Autodesk Inventor part; units mm, degrees
ref_plane "YZ Plane" through (0, 0, 0) normal (1, 0, 0) x (0, 1, 0)
ref_plane "XZ Plane" through (0, 0, 0) normal (0, 1, 0) x (-1, 0, 0)
ref_plane "XY Plane" through (0, 0, 0) normal (0, 0, 1) x (1, 0, 0)
sketch "Sketch1" plane through (0, 0, 0) normal (0, 0, 1) x (1, 0, 0)
  arc A0 (-37, 0) -> (37, 0) centre (0, 0) ccw
  line L0 (-51.8, 0) -> (51.8, 0) construction
  circle A1 centre (0, 0) radius 35 construction
  line L1 (-37, 0) -> (37, 0)
  dimension "d1" = 70
  dimension "d2" = 2
extrude "Extrusion1" add sketch "Sketch1" along normal blind 2
sketch "Sketch2" plane through (0, 0, 2) normal (0, 0, 1) x (1, 0, 0)
  arc A0 (-37, 0) -> (37, 0) centre (0, 0) ccw
  arc A1 (-35, 0) -> (35, 0) centre (0, 0) ccw
  line L0 (37, 0) -> (-37, 0)
  line L1 (-37, 0) -> (37, 0)
  dimension "d5" = 2
extrude "Extrusion2" add sketch "Sketch2" along normal blind 35 contours L0 A1 A0
ref_plane "Work Plane1" through (0, 0, 19.5) normal (0, 0, 1) x (1, 0, 0)
mirror "Mirror1" about plane through (0, 0, 19.5) normal (0, 0, 1) of "Extrusion1"
sketch "Sketch3" plane through (0, 0, 39) normal (0, 0, 1) x (1, 0, 0)
  circle A0 centre (0, 0) radius 21
  dimension "d8" = 42
extrude "Extrusion3" cut sketch "Sketch3" against normal blind 35
sketch "Sketch4" plane through (0, 0, 0) normal (1, 0, 0) x (0, 1, 0)
  line L0 (-4, 9.5) -> (-31, 9.5)
  line L1 (-31, 9.5) -> (-31, 29.5)
  line L2 (-31, 29.5) -> (-4, 29.5)
  line L3 (-4, 29.5) -> (-4, 9.5)
  line L4 (-44.4, 19.5) -> (7.4, 19.5) construction
  line L5 (0, 0) -> (0, 39) construction
  line L6 (-35, 37) -> (-35, 2) construction
  dimension "d11" = 20
  dimension "d12" = 4
  dimension "d13" = 4
extrude "Extrusion4" cut sketch "Sketch4" along normal through all both and the other way through all
sketch "Sketch5" plane through (0, 0, 0) normal (0, 1, 0) x (-1, 0, 0)
  line L0 (37, 0) -> (-37, 0)
  line L1 (0, -31.0583) -> (0, 50.6764) construction
  line L2 (-6, -3) -> (6, -3)
  line L3 (6, -3) -> (6, -5.2)
  line L4 (6, -5.2) -> (-6, -5.2)
  line L5 (-6, -5.2) -> (-6, -3)
  line L6 (-2.5, -5.2) -> (2.5, -5.2)
  line L7 (2.5, -5.2) -> (2.5, -11.2)
  line L8 (2.5, -11.2) -> (-2.5, -11.2)
  line L9 (-2.5, -11.2) -> (-2.5, -5.2)
  line L10 (0, -3) -> (0, -11.2) construction
  line L11 (-37, 0) -> (37, 0) construction
  line L12 (-13.75, 0) -> (13.75, 0)
  line L13 (13.75, 0) -> (13.75, -3)
  line L14 (13.75, -3) -> (-13.75, -3)
  line L15 (-13.75, -3) -> (-13.75, 0)
  dimension "d32" = 2.2
  dimension "d33" = 3.5
  dimension "d34" = 6
  dimension "d35" = 5
  dimension "d36" = 27.5
  dimension "d37" = 3
extrude "Extrusion5" add sketch "Sketch5" against normal blind 30
sketch "Sketch6" plane through (0, 0, 2) normal (0, 0, 1) x (1, 0, 0)
  line L0 (0, 0) -> (0, -21) construction
  arc A0 (-21, 0) -> (21, 0) centre (0, 0) ccw
  point P0 (0, -10.5)
hole "Hole1" at (0, -10.5, 2) direction (0, 0, -1) diameter 5.5 end through all counterbore diameter 10 counterbore depth 5
sketch "Sketch7" plane through (-2.5, -30, -11.2) normal (-1, 0, 0) x (0, 0, 1)
  line L0 (6, 30) -> (6, 0)
  line L1 (0, 30) -> (0, 20.6456)
  line L2 (0, 18.3544) -> (0, 0)
  line L3 (0, 15) -> (6, 15)
  line L4 (6, 15) -> (6, 24)
  line L5 (6, 24) -> (0, 24)
  line L6 (0, 24) -> (0, 15)
  line L7 (6, 18.3544) -> (0, 18.3544) construction
  line L8 (0, 19.5) -> (6, 19.5) construction
  line L9 (6, 15) -> (0, 9)
  line L10 (0, 15) -> (0, 9)
  line L11 (0, 20.6456) -> (6, 20.6456) construction
  point P0 (11.2, 30)
  point P1 (0, 24)
  dimension "d39" = 9
  dimension "d41" = 1.1456
  dimension "d42" = 45
  dimension "d45" = 1.1456
extrude "Extrusion6" cut sketch "Sketch7" along normal through all both and the other way through all
equation "\"d13\" = d12"
equation "\"d45\" = d41"
properties part number "Winddingshalter"
CAD build for the part. Positions are in the model's coordinates, mm. A direction names the side the tool comes from. Give positions to 0.01 mm unless a question says otherwise; leave off trailing zeros. Loops run counter-clockwise (first coordinate to the right, second up) from the corner with the lowest first, then second, coordinate; pieces in that order, holes last. Notation, with made-up numbers: M 25,4.5 L 46,4.5 A30 ccw 46,38.5 Z; hole C 35,5.5 d3. An arc over 180 degrees is marked long. One line per question, with ' | ' between items. Start each with the question number.
1. Probe L1, parallel to Z at x = -24, y = -14.5; L2, parallel to Y at x = 0, z = -4.35; L3, parallel to Y at x = 0, z = 0.9. List the from-to ranges inside material, lowest first. Write a range as from..to.
2. Saw through at A-A on z = 11. Give the cut face in (x, y), plus the area to 3 significant figures.
3. Two-plate mould, pull along X, no slides. Class faces 5 (the face through (-0.1, -14.8, -5.2)), 6 (the face through (6, -15, -4)), 7 (the face through (-1.5, -15.27, -0.54)): pulls with the +X half, pulls with the -X half, needs draft (parallel to the pull), parting line crosses it, or undercut.
4. Flat gauge pins, fed straight in: pin 1 (0.7 mm diameter, centred on y = -17, z = -4.5, fed in from +X); pin 2 (2 mm diameter, centred on y = -21.5, z = 6.5, fed in from +X); pin 3 (10 mm diameter, centred on x = -23, z = 31, fed in from +Y); pin 4 (4 mm diameter, centred on y = -9.5, z = 26.5, fed in from -X). Where does each tip first touch, or does it go through?
5. Saw through at B-B on x = 0. Give the cut face in (y, z).
6. Saw through at D-D on y = -19.5. State how many separate pieces and enclosed holes the cut face has, plus the area to 3 significant figures.
7. Saw through at C-C on y = -29. Give the cut face in (x, z), plus the area to 3 significant figures.
8. 3-axis set-ups, long thin cutter, end or side, ignore diameter. For faces 1 (the face through (-2.5, -3, -8)), 2 (the face through (36, -4, 20)), 3 (the face through (0, -17, 2)), 4 (the face through (0, -30, -3)): which of +Z, -Z, +X, -X, +Y, -Y reach the whole face in a straight line?
Result sheet:
1) L1: z = 0..2, 37..39 | L2: y = -30..-13.25, -7.75..0 | L3: y = -37..-15.5, -5.5..0
2) outline: M -37,0 A37 ccw -36.78,-4 L -34.77,-4 A35 cw -35,0 Z; M -20.2,-31 A37 ccw 20.2,-31 L 16.25,-31 A35 cw -16.25,-31 Z; M 34.77,-4 L 36.78,-4 A37 ccw 37,0 L 35,0 A35 cw Z | area: 92.7 mm^2
3) face 5: needs draft | face 6: pulls with the +X half | face 7: undercut
4) pin 1: stops at x = 6 | pin 2: stops at x = 30.8 | pin 3: stops at y = -21 | pin 4: passes through
5) outline: M -37,0 L -30,0 L -30,-11.2 L -21,-11.2 L -15,-5.2 L -13.25,-5.2 L -13.25,-3 L -15.5,-3 L -15.5,2 L -35,2 L -35,37 L -21,37 L -21,39 L -37,39 Z; M -7.75,-5.2 L -6,-5.2 L -6,-11.2 L 0,-11.2 L 0,2 L -5.5,2 L -5.5,-3 L -7.75,-3 Z
6) separate pieces: 3 | enclosed holes: 0 | area: 423 mm^2
7) outline: M -22.98,0 L -13.75,0 L -13.75,-3 L -6,-3 L -6,-5.2 L -2.5,-5.2 L -2.5,-11.2 L 2.5,-11.2 L 2.5,-5.2 L 6,-5.2 L 6,-3 L 13.75,-3 L 13.75,0 L 22.98,0 L 22.98,9.5 L 19.6,9.5 L 19.6,2 L -19.6,2 L -19.6,9.5 L -22.98,9.5 Z; M -22.98,29.5 L -19.6,29.5 L -19.6,37 L 19.6,37 L 19.6,29.5 L 22.98,29.5 L 22.98,39 L -22.98,39 Z | area: 424 mm^2
8) face 1: -Z, -X, +Y, -Y | face 2: +X, -X, -Y | face 3: +Y | face 4: -Z, +X, -X, -Y
